The listing builds one solid part. Answer for the finished solid, in the listing's coordinates (mm). Face numbers are marked on the shaded views. A direction names the side the tool comes from. Give positions to 0.01 mm unless a question says otherwise; leave off trailing zeros. Loops run counter-clockwise (first coordinate to the right, second up) from the corner with the lowest first, then second, coordinate; pieces in that order, holes last. Notation, with made-up numbers: M -3.75,-20 L 11.25,-20 A29 ccw 11.25,19 Z; hole C 16,85 d5. An arc over 180 degrees is marked long. Use one line per item in the form item = value. Start each with the question number.
1. For the marked faces 5, 6, 7 and 8, determine the directions among +Z, -Z, +X, -X, +Y, -Y from which every point of the face is accessible in a straight line to the end or side of a thin tool.
2. Straight lines are drawn through the part: line 1 (Z direction, x = -0.25, y = 0); line 2 (Z direction, x = -6.5, y = -2); line 3 (Z direction, x = -2, y = 0). For each, find the intervals that lie inside material, in ascending order. Write a range as from..to.
3. Each of these flat-tipped pins is pushed along its axis until it touches: pin 1 Ø1.3 at (y, z) = (0.5, 27) entering from +X; pin 2 Ø6.5 at (x, y) = (-5.5, -1.5) entering from -Z; pin 3 Ø3 at (x, y) = (7.5, 0.5) entering from -Z; pin 4 Ø5 at (y, z) = (0, -11.43) entering from -X (3 decimals). Where does it stop, or does it pass through?
4. The part is cut by section A-A (y = 0). Write down the section's boundary in (x, z) (1 decimal).
5. The mould has two halves that part along Z. Classify the marked faces 1, 2, 3 and 4: released by +Z, released by -Z, zero draft, split by the parting line, or undercut.
6. The part is cut by section C-C (y = 4.5). Write down the section's boundary in (x, z) (1 decimal), and give its area (3 significant figures).
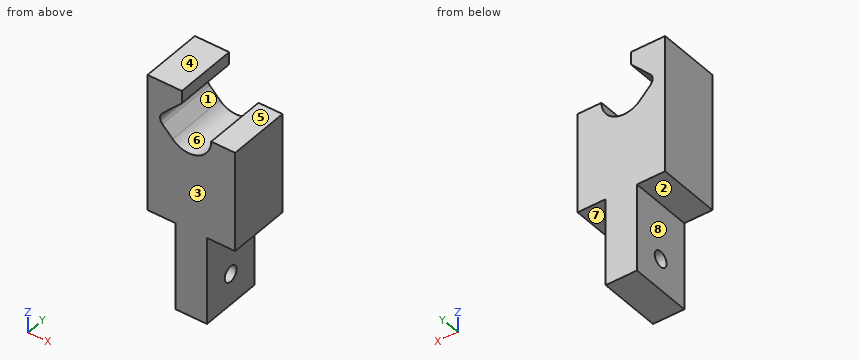
from build123d import *

# Parameters (mm, degrees)
F1_DEPTH = 6.35
F2_R     = 1.5875
F3_DEPTH = 12.066


with BuildPart() as f1:
    # F0 (on Front) → F1 (new body, symmetric)
    with BuildSketch(Plane.XZ):
        with BuildLine():
            Line((-3.175, -17.78), (3.175, -17.78))
            Line((3.175, -17.78), (3.175, 0))
            Line((3.175, 0), (8.89, 0))
            Line((8.89, 0), (8.89, 20.32))
            Line((8.89, 20.32), (4.03022, 20.32))
            ThreePointArc((4.03022, 20.32), (1.207849, 16.096023), (-3.774672, 17.087108))
            Line((-3.774672, 17.087108), (-5.885032, 19.197468))
            ThreePointArc((-5.885032, 19.197468), (-6.35, 20.32), (-5.885032, 21.442532))
            Line((-5.885032, 21.442532), (-1.927564, 25.4))
            Line((-1.927564, 25.4), (-1.927564, 27.94))
            Line((-1.927564, 27.94), (-8.89, 27.94))
            Line((-8.89, 27.94), (-8.89, 0))
            Line((-8.89, 0), (-3.175, 0))
            Line((-3.175, 0), (-3.175, -17.78))
        make_face()
    extrude(amount=F1_DEPTH, both=True)

    # F2 (on face) → F3 (cut, through all)
    with BuildSketch(Plane(origin=(-3.175, 0, 0), x_dir=(0, -1, 0), z_dir=(-1, 0, 0))):
        with Locations((0, -11.43)):
            Circle(F2_R)
    extrude(amount=-F3_DEPTH, mode=Mode.SUBTRACT)


solid = f1.part
Derived:
q1.face_5 = +Z, +X, +Y, -Y
q1.face_6 = +Y, -Y
q1.face_7 = -Z, +X, +Y, -Y
q1.face_8 = -Z, -X, +Y, -Y
q2.line_1 = -17.78..-13.02, -9.84..15.76
q2.line_2 = 0..27.94
q2.line_3 = -17.78..-13.02, -9.84..15.99, 25.33..27.94
q3.pin_1 = -1.93
q3.pin_2 = -17.78
q3.pin_3 = 0
q3.pin_4 = -3.175
q4.outline = M -8.9,0 L -3.2,0 L -3.2,-9.8 L 3.2,-9.8 L 3.2,0 L 8.9,0 L 8.9,20.3 L 4,20.3 A4.6 cw -3.8,17.1 L -5.9,19.2 A1.6 cw -5.9,21.4 L -1.9,25.4 L -1.9,27.9 L -8.9,27.9 Z; M -3.2,-17.8 L 3.2,-17.8 L 3.2,-13 L -3.2,-13 Z
q5.face_1 = undercut
q5.face_2 = released by -Z
q5.face_3 = zero draft
q5.face_4 = released by +Z
q6.outline = M -8.9,0 L -3.2,0 L -3.2,-17.8 L 3.2,-17.8 L 3.2,0 L 8.9,0 L 8.9,20.3 L 4,20.3 A4.6 cw -3.8,17.1 L -5.9,19.2 A1.6 cw -5.9,21.4 L -1.9,25.4 L -1.9,27.9 L -8.9,27.9 Z
q6.area = 480 mm2
